Build history of the part. All positions in model axes, mm. A direction names the side the tool comes from. Round coordinates to 2 decimals unless told otherwise and drop trailing zeros. Order: outer loops, then holes, each group sorted by start corner. A loop starts at its lowest first (then second) coordinate and runs counter-clockwise, first axis right, second up. Notation, with made-up numbers: (78, 9.5) - (124, 9.5) arc R6 ccw to (124, 19.5) - close; hole circle Ø7 at (-19, 74.5). An arc over 180 degrees is marked (long way). One line per question, with ' | ' between items. Start each with the question number.
Autodesk Inventor part; units mm, degrees
ref_plane "Work Plane1" through (20.15, 10, -1.65) normal (-1, 0, 0) x (0, 1, 0)
ref_plane "YZ Plane" through (0, 0, 0) normal (1, 0, 0) x (0, 1, 0)
ref_plane "XZ Plane" through (0, 0, 0) normal (0, 1, 0) x (-1, 0, 0)
sketch "Sketch1" plane through (0, 0, 0) normal (0, 0, 1) x (1, 0, 0)
  line L0 (0, 0) -> (-6.8, 0)
  line L1 (-6.8, 0) -> (-6.8, 20)
  line L2 (-6.8, 20) -> (0, 20)
  line L3 (0, 20) -> (0, 0)
  line L4 (-5.8439, 5.5) -> (-6.8, 5.5)
  line L5 (-6.8, 14.5) -> (-6.8, 5.5)
  line L6 (-6.8, 14.5) -> (-5.8439, 14.5)
  arc A0 (-5.8439, 14.5) -> (-5.8439, 16.9) centre (-4, 15.7) ccw
  line L7 (-5.8439, 16.9) -> (-6.8, 16.9)
  line L8 (-6.8, 20) -> (-6.8, 16.9)
  line L9 (0, 20) -> (-6.8, 20)
  line L10 (0, 0) -> (0, 20)
  line L11 (0, 0) -> (-6.8, 0)
  line L12 (-6.8, 3.1) -> (-6.8, 0)
  line L13 (-6.8, 3.1) -> (-5.8439, 3.1)
  arc A1 (-5.8439, 3.1) -> (-5.8439, 5.5) centre (-4, 4.3) ccw
  dimension "d0" = 6.8
  dimension "d1" = 20
extrude "Extrusion1" add sketch "Sketch1" along normal blind 5 contours L0 L1 L13 A1 L4 L6 A0 L7 L2 L3
ref_plane "Work Plane1" through (20.15, 10, -1.65) normal (-1, 0, 0) x (0, 1, 0)
mirror "Mirror1" about plane through (20.15, 10, -1.65) normal (-1, 0, 0) of "Extrusion1"
sketch "Sketch2" plane through (-6.8, 0, 0) normal (0, -1, 0) x (1, 0, 0)
  line L0 (0, 0) -> (53.9, 0)
  line L1 (53.9, 0) -> (53.9, 5)
  line L2 (53.9, 5) -> (0, 5)
  line L3 (0, 5) -> (0, 0)
  dimension "d4" = 53.9
extrude "Extrusion2" add sketch "Sketch2" along normal blind 5
sketch "Sketch3" plane through (-6.8, 3.1, 0) normal (-1, 0, 0) x (0, 0, 1)
  line L0 (0, -8.1) -> (5, -8.1)
  line L1 (5, -8.1) -> (5, 16.9)
  line L2 (5, 16.9) -> (0, 16.9)
  line L3 (0, 16.9) -> (0, -8.1)
  point P0 (0, -3.1)
  dimension "d7" = 25
extrude "Extrusion3" add sketch "Sketch3" along normal blind 2
mirror "Mirror2" about plane through (20.15, 10, -1.65) normal (-1, 0, 0) of "Extrusion3"
fillet "Fillet1" radius 2 1 edges at (-8.8, -5, 2.5)
fillet "Fillet2" radius 2 1 edges at (49.1, -5, 2.5)
sketch "Sketch4" plane through (0, 20, 5) normal (1, 0, 0) x (0, 0, -1)
  line L0 (5, -20) -> (5, 0)
  line L1 (5, 0) -> (0, 0)
  line L2 (0, -20) -> (0, 0)
  line L3 (5, -20) -> (0, -20)
extrude "Extrusion4" cut sketch "Sketch4" against normal blind 0.25
mirror "Mirror3" about plane through (20.15, 10, -1.65) normal (-1, 0, 0) of "Extrusion4"
sketch "Sketch5" plane through (-8.8, 20, 5) normal (0, 1, 0) x (1, 0, 0)
  line L0 (0, 0) -> (57.9, 0)
  line L1 (57.9, 0) -> (57.9, 5)
  line L2 (57.9, 5) -> (0, 5)
  line L3 (0, 5) -> (0, 0)
  point P0 (8.8, 5)
  dimension "d14" = 57.9
extrude "Extrusion5" add sketch "Sketch5" along normal blind 5
sketch "Sketch6" plane through (-8.8, 20, 5) normal (0, -1, 0) x (1, 0, 0)
  line L0 (8.55, 0) -> (8.55, -5)
  line L1 (49.35, -5) -> (8.55, -5)
  line L2 (49.35, -5) -> (49.35, 0)
  line L3 (8.55, 0) -> (49.35, 0)
  point P0 (8.8, -5)
extrude "Extrusion6" cut sketch "Sketch6" against normal blind 0.15
sketch "Sketch7" plane through (-6.8, 0, 0) normal (0, 1, 0) x (1, 0, 0)
  line L0 (47.35, -5) -> (6.55, -5)
  line L1 (47.35, 0) -> (47.35, -5)
  line L2 (6.55, 0) -> (47.35, 0)
  line L3 (6.55, 0) -> (6.55, -5)
  point P0 (6.8, 0)
extrude "Extrusion7" cut sketch "Sketch7" against normal blind 0.15
sketch "Sketch16" plane through (-8.8, 25, 5) normal (0, 1, 0) x (1, 0, 0)
  line L0 (0, 0) -> (57.9, 0)
  line L1 (0, 5) -> (15, 5)
  line L2 (15, 5) -> (15, 0)
  line L3 (15, 0) -> (0, 0)
  line L4 (0, 0) -> (0, 5)
  line L5 (57.9, 5) -> (42.9, 5)
  line L6 (42.9, 5) -> (42.9, 0)
  line L7 (42.9, 0) -> (57.9, 0)
  line L8 (57.9, 0) -> (57.9, 5)
  point P0 (8.8, 5)
  dimension "d48" = 15
  dimension "d49" = 15
extrude "Extrusion13" add sketch "Sketch16" along normal blind 18
sketch "Sketch17" plane through (0, 0, 0) normal (0, 0, -1) x (-1, 0, 0)
  line L0 (8.8, -3) -> (8.8, 43)
  line L1 (-34.1, 25) -> (-34.1, 43)
  line L2 (-49.1, 43) -> (-49.1, -3)
  line L3 (-49.1, 43) -> (-34.1, 43)
  line L4 (-34.1, 38) -> (-34.1, 36.5)
  line L5 (-49.1, 36.5) -> (-49.1, 43)
  line L6 (-6.2, 43) -> (8.8, 43)
  line L7 (8.8, 43) -> (8.8, 38)
  line L8 (8.8, 38) -> (-6.2, 38)
  line L9 (-6.2, 38) -> (-6.2, 43)
  line L10 (-49.1, 28.15) -> (-34.1, 28.15)
  line L11 (-34.1, 28.15) -> (-34.1, 21.65)
  line L12 (-34.1, 21.65) -> (-49.1, 21.65)
  line L13 (-49.1, 21.65) -> (-49.1, 28.15)
  line L14 (-6.2, 25) -> (8.8, 25)
  line L15 (8.8, 25) -> (8.8, 30)
  line L16 (8.8, 30) -> (-6.2, 30)
  line L17 (-6.2, 30) -> (-6.2, 25)
  line L18 (-40.55, 20.15) -> (0.25, 20.15)
  line L19 (-49.1, 36.15) -> (-34.1, 36.15)
  line L20 (-34.1, 36.15) -> (-34.1, 42.65)
  line L21 (-34.1, 42.65) -> (-49.1, 42.65)
  line L22 (-49.1, 42.65) -> (-49.1, 36.15)
  point P0 (0, 0)
  dimension "d54" = 6.5
  dimension "d75" = 1.5
  dimension "d76" = 8
  dimension "d77" = 6.5
sketch "Sketch19" plane through (-8.8, 25, 5) normal (0, 1, 0) x (1, 0, 0)
  line L0 (15, 5) -> (15, 0)
  line L1 (15, 0) -> (42.9, 0)
  line L2 (42.9, 0) -> (42.9, 5)
  line L3 (42.9, 5) -> (15, 5)
  point P0 (8.8, 5)
extrude "Extrusion17" add sketch "Sketch19" along normal up to surface (18 mm away)
extrude "Extrusion18" add sketch "Sketch17" along normal blind 30 contours L11 L12 L2 L10 L1 | L19 L2 L21 L1
fillet "Fillet16" radius 5 4 edges at (49.1, 39.4, -30) (34.1, 39.4, -30) (34.1, 24.9, -30) (49.1, 24.9, -30)
mirror "Mirror6" about plane through (20.15, 10, -1.65) normal (-1, 0, 0) of "Extrusion18", "Mirror1"
sketch "Sketch20" plane through (-8.8, 43, 5) normal (0, 1, 0) x (1, 0, 0)
  line L0 (57.9, 5) -> (0, 5)
  line L1 (0, 5) -> (0, 0)
  line L2 (0, 0) -> (57.9, 0)
  line L3 (57.9, 0) -> (57.9, 5)
  point P0 (8.8, 5)
extrude "Extrusion19" cut sketch "Sketch20" against normal up to surface (0.35 mm away)
mirror "Mirror7" about plane through (20.15, 10, -1.65) normal (-1, 0, 0) of "Fillet16"
ref_plane "Work Plane2" through (20.15, 10, -1.65) normal (-1, 0, 0) x (0, 1, 0)
ref_plane "Work Plane3" through (20.15, 10, -1.65) normal (-1, 0, 0) x (0, 1, 0)
properties part number "CameraCraddle"
Item 1: Slice it at A-A (y = 4.3). Write the cut outline in (x, z), plus the area to 4 significant figures.
Item 2: Slice it at B-B (z = -8). Write the cut outline in (x, y).
Item 3: Pin check, flat tips, straight feed: pin 1 (7 mm diameter, centred on x = 44.3, y = 4.3, fed in from -Z); pin 2 (4.5 mm diameter, centred on x = -2, z = -21, fed in from -Y). Stop position of each tip, or through.
Item 4: Wall check: line 1 along X through (y, z) = (15.7, 1.45); line 2 along Y through (x, z) = (-4, 1.55); line 3 along Y through (x, z) = (37.5, -27.5). Give the ranges that are in metal, low to high. Write a range as [from, to].
Item 5: Pull direction X, two halves, no side cores. Call faces 6 (the face through (35.53, 24.85, -28.5)), 7 (the face through (-1, 39, -30)), 8 (the face through (47.67, 39.45, -28.5)), 9 (the face through (-8.23, -4.4, 2.54)): released by +X, released by -X, zero draft, split by the parting line, or undercut.
Item 6: Slice it at D-D (z = 3.5). Count the separate pieces of the cut face and the enclosed holes in it, plus the area to 3 significant figures.
Item 7: 3-axis set-ups, long thin cutter, end or side, ignore diameter. For faces 1 (the face through (-6.8, 4, 2)), 2 (the face through (-1, 36.15, -15)), 3 (the face through (20, -5, 3)), 4 (the face through (34.1, 39, -12)), 5 (the face through (41, 21.65, -15)): which of +Z, -Z, +X, -X, +Y, -Y reach the whole face in a straight line?
Item 8: Slice it at C-C (x = 33). Write the cut outline in (y, z), plus the area to 3 significant figures.
A:
1) outline: (-8.8, 0) - (-6.8, 0) - (-6.8, 5) - (-8.8, 5) - close; (-1.8, 0) - (0, 0) - (0, 5) - (-1.8, 5) - close; (40.55, 0) - (42.1, 0) - (42.1, 5) - (40.55, 5) - close; (47.1, 0) - (49.1, 0) - (49.1, 5) - (47.1, 5) - close | area: 36.75 mm^2
2) outline: (-8.8, 21.65) - (6.2, 21.65) - (6.2, 28.15) - (-8.8, 28.15) - close; (-8.8, 36.15) - (6.2, 36.15) - (6.2, 42.65) - (-8.8, 42.65) - close; (34.1, 21.65) - (49.1, 21.65) - (49.1, 28.15) - (34.1, 28.15) - close; (34.1, 36.15) - (49.1, 36.15) - (49.1, 42.65) - (34.1, 42.65) - close
3) pin 1: z = 0 | pin 2: y = 21.65
4) line 1: [-8.8, -6.8], [-1.8, 0], [40.55, 42.1], [47.1, 49.1] | line 2: [-5, 2.1], [6.5, 13.5], [17.9, 42.65] | line 3: [21.65, 28.15], [36.15, 42.65]
5) face 6: undercut | face 7: zero draft | face 8: released by +X | face 9: released by -X
6) separate pieces: 1 | enclosed holes: 5 | area: 1,870 mm^2
7) face 1: +Z, -Z | face 2: -Z, +X, -X | face 3: +Z, -Z, +X, -X, -Y | face 4: -Z, +Y, -Y | face 5: -Z, +X, -X, -Y
8) outline: (-5, 0) - (-0.15, 0) - (-0.15, 5) - (-5, 5) - close; (20.15, 0) - (42.65, 0) - (42.65, 5) - (20.15, 5) - close | area: 137 mm^2
